from build123d import *

# Parameters (mm, degrees)
BOSS_EXTRUDE1_DEPTH = 7
SKETCH2_R           = 3
CUT_EXTRUDE1_DEPTH  = 14
FILLET1_R           = 0.5


with BuildPart() as part:
    # Sketch1 → Boss-Extrude1 (new, symmetric)
    with BuildSketch(Plane.XY):
        with BuildLine():
            Line((-40, 0), (40, 0))
            Line((40, 0), (36.78663137, 12.715119427))
            ThreePointArc((36.78663137, 12.715119427), (34.30082341, 16.522944685), (30, 18))
            Line((30, 18), (30, 10))
            Line((30, 10), (-30, 10))
            Line((-30, 10), (-30, 18))
            ThreePointArc((-30, 18), (-34.30082341, 16.522944685), (-36.78663137, 12.715119427))
            Line((-36.78663137, 12.715119427), (-40, 0))
        make_face()
    extrude(amount=BOSS_EXTRUDE1_DEPTH, both=True)

    # Sketch2 → Cut-Extrude1 (cut)
    with BuildSketch(Plane(origin=(0, 10, 0), x_dir=(1, 0, 0), z_dir=(0, 1, 0))):
        with Locations(Location((-23, 0, 0), (0, 0, 270))):
            Circle(SKETCH2_R)
        with Locations(Location((22, 0, 0), (0, 0, 270))):
            Circle(SKETCH2_R)
    extrude(amount=-CUT_EXTRUDE1_DEPTH, mode=Mode.SUBTRACT)

    # Fillet1
    fillet1_edges = [part.edges().sort_by_distance(p)[0] for p in [
        (34.30082341, 16.522944685, -7),
        (38.393315685, 6.357559714, -7),
        (0, 0, -7),
        (-38.393315685, 6.357559714, -7),
        (38.393315685, 6.357559714, 7),
        (-30, 18, 0),
        (-30, 10, 0),
        (40, 0, 0),
        (34.30082341, 16.522944685, 7),
        (30, 14, 7),
        (0, 10, 7),
        (-30, 14, 7),
        (-34.30082341, 16.522944685, 7),
        (-38.393315685, 6.357559714, 7),
        (-34.30082341, 16.522944685, -7),
        (0, 0, 7),
        (-30, 14, -7),
        (0, 10, -7),
        (30, 14, -7),
    ]]
    fillet(fillet1_edges, radius=FILLET1_R)


solid = part.part
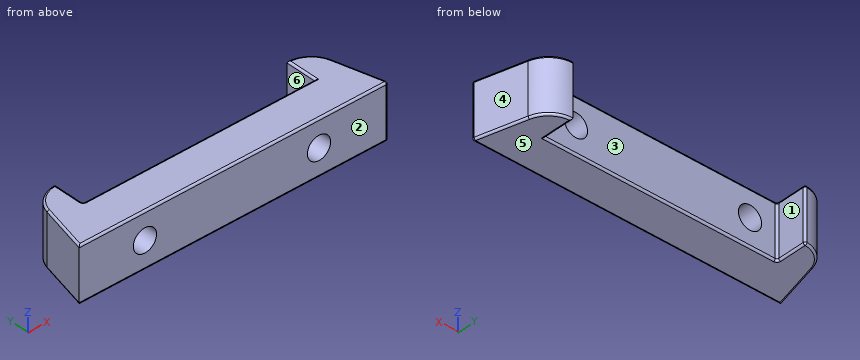
Could you check a few things on this model? Use its own coordinates, in mm. Face numbers are marked on the shaded views. A direction names the side the tool comes from. Coordinates: 2 decimals unless noted, no trailing zeros. Write each loop counter-clockwise with the first axis right and the second up, starting at its lowest first coordinate (ties: lowest second). Pieces come first, ordered by that corner, then holes. Notation, with made-up numbers: (25, -16.75) - (35, -16.75) arc R27 ccw to (35, -0.75) - close; hole circle Ø7 at (12, 6.5). An arc over 180 degrees is marked (long way). Put each result on its own line as item: value. Start each with the question number.
Q1. I'm going to push flat-ended pins straight in: P1, Ø4, axis at y = 14.5, z = -1, coming from the -X side; P2, Ø6.5, axis at x = -8, z = 0, coming from the +Y side; P3, Ø3, axis at y = 3.5, z = -3, coming from the -X side. Where does each tip first touch, or does it pass through?
Q2. I want a section at A-A on x = 22. Write out the boundary of the cut face in (y, z).
Q3. I want a section at B-B on z = -1.75. Write out the boundary of the cut face in (x, y), plus the area to 3 significant figures.
Q4. I want a section at D-D on x = -16.5. Write out the boundary of the cut face in (y, z).
Q5. Thinking about a two-plate mould opening in X: for the marked faces 1, 2, 3 and 4, which applies, pulls with the +X half, pulls with the -X half, needs draft (parallel to the pull), parting line crosses it, or undercut?
Q6. Please list where these lines run through material, in increasing order: L1, parallel to X at y = 3.25, z = 0; L2, parallel to X at y = 3.75, z = 0; L3, parallel to Y at x = 20.5, z = 5.
Q7. Which directions (+Z, -Z, +X, -X, +Y, -Y) give clear straight access to the entire face, cutting with the end or side of a thin tool? Please do the marked faces 5 and 6.
Q8. I want a section at C-C on z = 5.75. Write out the boundary of the cut face in (x, y).
Checks:
1. P1: x = -36.84
1. P2: y = 10
1. P3: x = -39.49
2. outline: (0, -6.5) arc R0.5 ccw to (0.5, -7) - (9.5, -7) arc R0.5 ccw to (10, -6.5) - (10, -3) - (0, -3) - close; (0, 3) - (10, 3) - (10, 6.5) arc R0.5 ccw to (9.5, 7) - (0.5, 7) arc R0.5 ccw to (0, 6.5) - close
3. outline: (-40, 0) - (-25.44, 0) - (-25.44, 10) - (-29.5, 10) arc R0.5 cw to (-30, 10.5) - (-30, 17.48) arc R0.5 ccw to (-30.54, 17.98) arc R7 ccw to (-36.79, 12.72) - close; (-20.56, 0) - (19.56, 0) - (19.56, 10) - (-20.56, 10) - close; (24.44, 0) - (39.36, 0) arc R0.5 ccw to (39.84, 0.62) - (36.79, 12.72) arc R7 ccw to (30, 18) - (30, 10) - (24.44, 10) - close
3. area: 769 mm²
4. outline: (0, -6.5) arc R0.5 ccw to (0.5, -7) - (9.5, -7) arc R0.5 ccw to (10, -6.5) - (10, 6.5) arc R0.5 ccw to (9.5, 7) - (0.5, 7) arc R0.5 ccw to (0, 6.5) - close
5. face 1: undercut
5. face 2: needs draft
5. face 3: undercut
5. face 4: pulls with the +X half
6. L1: -39.18 to -26, -20 to 19, 25 to 39.18
6. L2: -39.05 to -26, -20 to 19, 25 to 39.05
6. L3: 0 to 10
7. face 5: -Z, +X, -X, +Y, -Y
7. face 6: +Z, -Z, +Y
8. outline: (-40, 0) - (39.36, 0) arc R0.5 ccw to (39.84, 0.62) - (36.79, 12.72) arc R7 ccw to (30, 18) - (30, 10) - (-29.5, 10) arc R0.5 cw to (-30, 10.5) - (-30, 17.48) arc R0.5 ccw to (-30.54, 17.98) arc R7 ccw to (-36.79, 12.72) - close
